Verification items for the finished model (mm, model axes). Face numbers are marked on the shaded views. A direction names the side the tool comes from. Round coordinates to 2 decimals unless told otherwise and drop trailing zeros. Write each loop counter-clockwise with the first axis right and the second up, starting at its lowest first coordinate (ties: lowest second). Pieces come first, ordered by that corner, then holes. Notation, with made-up numbers: M 31,69.25 L 38,69.25 A23 ccw 38,79.25 Z; hole C 80,66.25 d4. An arc over 180 degrees is marked long. One line per question, with ' | ' between items.
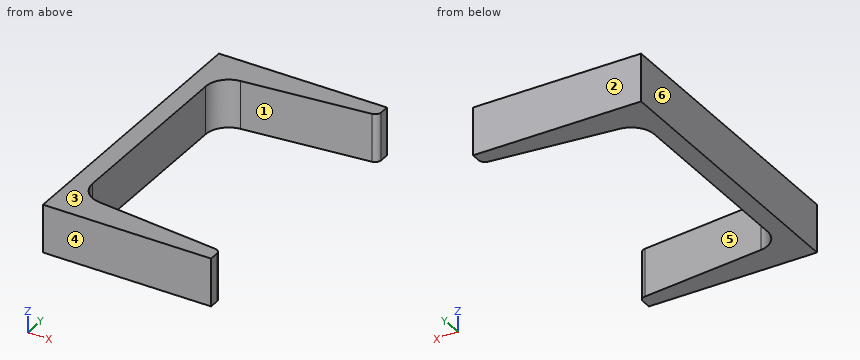
from build123d import *

# Parameters (mm, degrees)
BASEMCHANNEL_DEPTH = 12.7
TOEFILLET_R        = 3.175


with BuildPart() as part:
    # Sketch1 → BaseMchannel (new body, symmetric)
    with BuildSketch(Plane.XY):
        with BuildLine():
            Line((89.0016, 152.4), (0, 152.4))
            Line((0, 152.4), (0, 0))
            Line((0, 0), (89.0016, 0))
            Line((89.0016, 0), (89.0016, 7.893675663))
            Line((89.0016, 7.893675663), (20.544188976, 15.088839497))
            ThreePointArc((20.544188976, 15.088839497), (12.758178288, 19.056010093), (9.6266, 27.214050446))
            Line((9.6266, 27.214050446), (9.6266, 125.185949554))
            ThreePointArc((9.6266, 125.185949554), (12.758178288, 133.343989907), (20.544188976, 137.311160503))
            Line((20.544188976, 137.311160503), (89.0016, 144.506324337))
            Line((89.0016, 144.506324337), (89.0016, 152.4))
        make_face()
    extrude(amount=BASEMCHANNEL_DEPTH, both=True)

    # ToeFillet
    toefillet_edges = [part.edges().sort_by_distance(p)[0] for p in [
        (89.0016, 144.506324337, 0),
        (89.0016, 7.893675663, 0),
    ]]
    fillet(toefillet_edges, radius=TOEFILLET_R)


solid = part.part
1. Go/stop test with flat-tipped pins: P1, Ø5, axis at x = 44, z = 8, coming from the -Y side; P2, Ø1, axis at y = 38, z = 2.5, coming from the +X side. Record where each tip stops, or that it passes through.
Results:
P1: stops at y = 0 | P2: stops at x = 9.63
2. Section check C-C, the plane x = 59. Record the cut outline in (y, z), then the cut area to 3 significant figures.
Results:
outline: M 0,-12.7 L 11.05,-12.7 L 11.05,12.7 L 0,12.7 Z; M 141.35,-12.7 L 152.4,-12.7 L 152.4,12.7 L 141.35,12.7 Z | area: 561 mm2
3. Thickness scan on line 1 (X direction, y = 43, z = -0.5); line 2 (Y direction, x = 66.5, z = 0.5); line 3 (Y direction, x = 24.5, z = -6.75). Record the ranges inside material, lowest first.
Results:
line 1: x = 0 to 9.63 | line 2: y = 0 to 10.26, 142.14 to 152.4 | line 3: y = 0 to 14.67, 137.73 to 152.4
4. Tool access check on the marked faces 5 and 6. Record the directions out of +Z, -Z, +X, -X, +Y, -Y that give a thin tool (end or side, any length) a straight path to the whole face; none if there is none.
Results:
face 5: +Z, -Z, +X | face 6: +Z, -Z, -X, +Y, -Y
5. Mould release check, pull along Y, two halves, no side actions. Record for the marked faces 1, 2, 3 and 4: pulls with the +Y half, pulls with the -Y half, needs draft (parallel to the pull), parting line crosses it, or undercut.
Results:
face 1: undercut | face 2: pulls with the +Y half | face 3: needs draft | face 4: pulls with the -Y half
6. Section check A-A, the plane x = 78. Record the cut outline in (y, z).
Results:
outline: M 0,-12.7 L 9.05,-12.7 L 9.05,12.7 L 0,12.7 Z; M 143.35,-12.7 L 152.4,-12.7 L 152.4,12.7 L 143.35,12.7 Z
7. Section check D-D, the plane y = 89. Record the cut outline in (x, z), then the cut area to 3 significant figures.
Results:
outline: M 0,-12.7 L 9.63,-12.7 L 9.63,12.7 L 0,12.7 Z | area: 245 mm2
